The listing builds one solid part. Answer for the finished solid, in the listing's coordinates (mm). Face numbers are marked on the shaded views. A direction names the side the tool comes from. Give positions to 0.01 mm unless a question says otherwise; leave off trailing zeros. Loops run counter-clockwise (first coordinate to the right, second up) from the corner with the lowest first, then second, coordinate; pieces in that order, holes last. Notation, with made-up numbers: M -12.5,37 L 7.5,37 A26 cw 7.5,67 Z; hole C 23.25,9 d1. An arc over 180 degrees is marked long. Use one line per item in the form item = value. Start each with the question number.
1. The mould has two halves that part along X. Classify the marked faces 1 and 2: released by +X, released by -X, zero draft, split by the parting line, or undercut.
2. Straight lines are drawn through the part: line 1 (Y direction, x = -9, z = 0.75); line 2 (X direction, y = -8, z = 8.75); line 3 (Y direction, x = 26, z = 0.5). For each, find the intervals that lie inside material, in ascending order. Write a range as from..to.
3. The part is cut by section C-C (y = -5). Write down the section's boundary in (x, z).
4. For the marked faces 3, 4 and 5, determine the directions among +Z, -Z, +X, -X, +Y, -Y from which every point of the face is accessible in a straight line to the end or side of a thin tool.
5. Each of these flat-tipped pins is pushed along its axis until it touches: pin 1 Ø6 at (x, y) = (-9.5, -14) entering from +Z; pin 2 Ø0.6 at (x, z) = (-17, 8) entering from +Y; pin 3 Ø4 at (x, y) = (26, -11.5) entering from +Z. Where does it stop, or does it pass through?
6. The part is cut by section B-B (z = 7.5). Write down the section's boundary in (x, y).
7. The part is cut by section D-D (y = 9). Write down the section's boundary in (x, z).
from build123d import *

# Parameters (mm, degrees)
SKETCH_W        = 50
SKETCH_H        = 34.5
PAD_DEPTH       = 1.2
SKETCH001_R     = 2.6
POCKET_DEPTH    = 1.201
SKETCH002_W     = 1.2
SKETCH002_H     = 24.4
PAD001_DEPTH    = 10
SKETCH003_W     = 50
SKETCH003_H     = 14.1
PAD002_DEPTH    = 1.2
SKETCH004_R     = 2.6
SKETCH004_W     = 12.5
SKETCH004_H     = 2.5
POCKET001_DEPTH = 14.101
SKETCH005_R     = 4.6
SKETCH005_R_2   = 2.6
PAD003_DEPTH    = 1.2
FILLET_R        = 1
FILLET001_R     = 5
SKETCH006_R     = 3.8
SKETCH006_R_2   = 2.6
PAD004_DEPTH    = 6.9
SKETCH007_W     = 9
SKETCH007_H     = 2
SKETCH007_W_2   = 3.353744
SKETCH007_H_2   = 0.7
POCKET002_DEPTH = 10


with BuildPart() as part:
    # Sketch → Pad (new body)
    with BuildSketch(Plane.XY):
        Rectangle(SKETCH_W, SKETCH_H)
    extrude(amount=PAD_DEPTH)

    # Sketch001 (on Face6 of Pad) → Pocket (cut, through all)
    with BuildSketch(Plane.XY.offset(1.2)):
        with Locations((0, -14.85)):
            Circle(SKETCH001_R)
        with Locations((-19, 10.15)):
            Circle(SKETCH001_R)
        with Locations((13, 13.842333)):
            Circle(SKETCH001_R)
        with Locations((26, -12.638792)):
            Circle(SKETCH001_R)
    extrude(amount=-POCKET_DEPTH, mode=Mode.SUBTRACT)

    # Sketch002 (on Face5 of Pocket) → Pad001 (join)
    with BuildSketch(Plane.XY.offset(1.2)):
        with Locations((-3.5, -5.05)):
            Rectangle(SKETCH002_W, SKETCH002_H)
        with Locations((-17.2, -5.05)):
            Rectangle(SKETCH002_W, SKETCH002_H)
    extrude(amount=PAD001_DEPTH)

    # Sketch003 (on Face6 of Pad001) → Pad002 (join)
    with BuildSketch(Plane.XZ.offset(17.25)):
        with Locations((0, -5.85)):
            Rectangle(SKETCH003_W, SKETCH003_H)
    extrude(amount=-PAD002_DEPTH)

    # Sketch004 (on Face5 of Pad002) → Pocket001 (cut, through all)
    with BuildSketch(Plane.XY.offset(1.2)):
        with Locations((0, -14.85)):
            Circle(SKETCH004_R)
        with Locations((-10.35, -8.5)):
            Rectangle(SKETCH004_W, SKETCH004_H)
    extrude(amount=-POCKET001_DEPTH, mode=Mode.SUBTRACT)

    # Sketch005 (on Face5 of Pocket001) → Pad003 (join)
    with BuildSketch(Plane.XY.offset(1.2)):
        with Locations((26, -12.638792)):
            Circle(SKETCH005_R)
        with Locations((26, -12.638792)):
            Circle(SKETCH005_R_2, mode=Mode.SUBTRACT)
    extrude(amount=-PAD003_DEPTH)

    # Fillet
    fillet_edges = [part.edges().sort_by_distance(p)[0] for p in [
        (-25, -17.25, -6.45),
        (-25, -17.25, 0.6),
    ]]
    fillet(fillet_edges, radius=FILLET_R)

    # Fillet001
    fillet001_edges = [part.edges().sort_by_distance(p)[0] for p in [
        (-25, 17.25, 0.6),
        (25, 17.25, 0.6),
    ]]
    fillet(fillet001_edges, radius=FILLET001_R)

    # Sketch006 (on Face5 of Fillet001) → Pad004 (join)
    with BuildSketch(Plane.XY.offset(1.2)):
        with Locations((-19, 10.15)):
            Circle(SKETCH006_R)
        with Locations((-19, 10.15)):
            Circle(SKETCH006_R_2, mode=Mode.SUBTRACT)
        with Locations((12.996001, 13.84)):
            Circle(SKETCH006_R)
        with Locations((12.996001, 13.84)):
            Circle(SKETCH006_R_2, mode=Mode.SUBTRACT)
        with Locations((26, -12.638792)):
            Circle(SKETCH006_R)
        with Locations((26, -12.638792)):
            Circle(SKETCH006_R_2, mode=Mode.SUBTRACT)
        with Locations((0, -14.85)):
            Circle(SKETCH006_R)
        with Locations((0, -14.85)):
            Circle(SKETCH006_R_2, mode=Mode.SUBTRACT)
    extrude(amount=PAD004_DEPTH)

    # Sketch007 (on Face5 of Pad004) → Pocket002 (cut)
    with BuildSketch(Plane.XY.offset(1.2)):
        with Locations((0.4, -18.25)):
            Rectangle(SKETCH007_W, SKETCH007_H)
        with Locations((12.996001, 17.6)):
            Rectangle(SKETCH007_W_2, SKETCH007_H_2)
    extrude(amount=POCKET002_DEPTH, mode=Mode.SUBTRACT)


solid = part.part
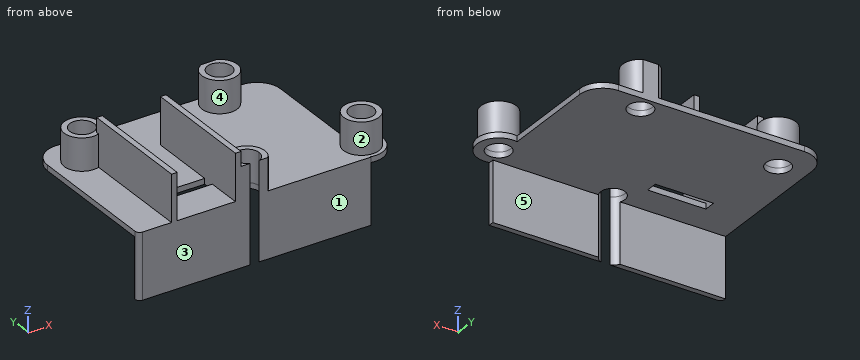
Derived:
q1.face_1 = zero draft
q1.face_2 = undercut
q2.line_1 = -17.25..-9.75, -7.25..17.25
q2.line_2 = -17.8..-16.6, -4.1..-2.9
q2.line_3 = -17.24..-15.24, -10.04..-8.04
q3.outline = M -25,0 L 25,0 L 25,1.2 L -2.9,1.2 L -2.9,11.2 L -4.1,11.2 L -4.1,1.2 L -16.6,1.2 L -16.6,11.2 L -17.8,11.2 L -17.8,1.2 L -25,1.2 Z
q4.face_3 = +Z, -Z, +X, -X, -Y
q4.face_4 = +Z
q4.face_5 = -Z, +X, -X, +Y
q5.pin_1 = 1.2
q5.pin_2 = 13.55
q5.pin_3 = 8.1
q6.outline = M -17.8,-17.25 L -16.6,-17.25 L -16.6,7.15 L -16.67,7.15 A3.8 ccw long -17.8,6.54 Z; M -4.1,-17.25 L -1,-17.25 A2.6 cw long 1,-17.25 L 2.95,-17.25 A3.8 ccw -2.9,-12.39 L -2.9,7.15 L -4.1,7.15 Z; M 11.32,17.25 A3.8 ccw long 14.67,17.25 Z; C 26,-12.64 d7.6; hole C -19,10.15 d5.2; hole C 13,13.84 d5.2; hole C 26,-12.64 d5.2
q7.outline = M -25,0 L -21.33,0 L -21.33,8.1 L -22.62,8.1 L -22.62,1.2 L -25,1.2 Z; M -16.67,0 L 25,0 L 25,1.2 L -15.38,1.2 L -15.38,8.1 L -16.67,8.1 Z
